Can you work these out from the model? Positions are in its coordinate system, mm. Face numbers are marked on the shaded views. A direction names the side the tool comes from. Round coordinates to 2 decimals unless told otherwise and drop trailing zeros. Order: outer loops, then holes, each group sorted by start corner. A loop starts at its lowest first (then second) coordinate and runs counter-clockwise, first axis right, second up. Notation, with made-up numbers: M 22,51 L 70,51 A25 ccw 70,84 Z; hole C -4,-35.75 d9. An arc over 180 degrees is marked long. One line per question, with ' | ' between items.
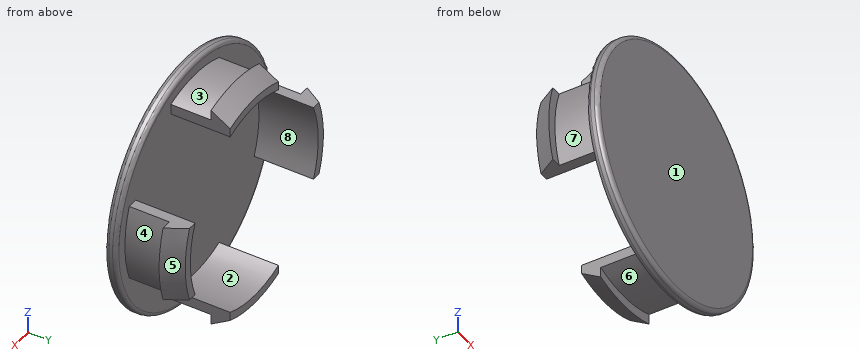
```python
from build123d import *

# Parameters (mm, degrees)
CUT_EXTRUDE_1_REACH = 51.545


with BuildPart() as part:
    # Эскиз1 → Повернуть1 (revolve)
    with BuildSketch(Plane.XY, mode=Mode.PRIVATE) as revolve_1_sk:
        with BuildLine():
            Line((0, 0), (-31.5, 0))
            ThreePointArc((-31.5, 0), (-32.207106781, 0.292893219), (-32.5, 1))
            Line((-32.5, 1), (-32.5, 2))
            ThreePointArc((-32.5, 2), (-32.207106781, 2.707106781), (-31.5, 3))
            Line((-31.5, 3), (-29, 3))
            Line((-29, 3), (-29, 13.5))
            Line((-29, 13.5), (-31.5, 13.5))
            Line((-31.5, 13.5), (-28.613248654, 18.5))
            Line((-28.613248654, 18.5), (-26.5, 18.5))
            Line((-26.5, 18.5), (-26.5, 3))
            Line((-26.5, 3), (0, 3))
            Line((0, 3), (0, 0))
        make_face()
    revolve(revolve_1_sk.sketch.rotate(Axis((0, 0, 0), (0, -1, 0)), 270), axis=Axis((0, 0, 0), (0, -1, 0)))

    # Вырез-Вытянуть1: up to this face of the body (flat: up to its plane)
    cut_extrude_1_end = Plane(part.part.faces().sort_by_distance((0, 3, -30.609045456))[0])
    # Эскиз2 → Вырез-Вытянуть1 (cut, up to the picked face)
    with BuildSketch(Plane(origin=(0, 18.5, 0), x_dir=(1, 0, 0), z_dir=(0, 1, 0)), mode=Mode.PRIVATE) as cut_extrude_1_sk1:
        with BuildLine():
            Line((-10, 26.8089164), (-10, 40.856644609))
            ThreePointArc((-10, 40.856644609), (-29.742775667, 29.742775667), (-40.856644609, 10))
            Line((-40.856644609, 10), (-26.8089164, 10))
            ThreePointArc((-26.8089164, 10), (-20.232622155, 20.232622155), (-10, 26.8089164))
        make_face()
    cut_extrude_1_tool1 = split(extrude(cut_extrude_1_sk1.sketch, amount=-CUT_EXTRUDE_1_REACH, mode=Mode.PRIVATE), bisect_by=cut_extrude_1_end, keep=Keep.BOTH, mode=Mode.PRIVATE)
    # Эскиз2 → Вырез-Вытянуть1 (cut, up to the picked face)
    with BuildSketch(Plane(origin=(0, 18.5, 0), x_dir=(1, 0, 0), z_dir=(0, 1, 0)), mode=Mode.PRIVATE) as cut_extrude_1_sk2:
        with BuildLine():
            ThreePointArc((26.8089164, 10), (20.232622155, 20.232622155), (10, 26.8089164))
            Line((10, 26.8089164), (10, 24.540782384))
            ThreePointArc((10, 24.540782384), (18.738329701, 18.738329701), (24.540782384, 10))
            Line((24.540782384, 10), (26.8089164, 10))
        make_face()
    cut_extrude_1_tool2 = split(extrude(cut_extrude_1_sk2.sketch, amount=-CUT_EXTRUDE_1_REACH, mode=Mode.PRIVATE), bisect_by=cut_extrude_1_end, keep=Keep.BOTH, mode=Mode.PRIVATE)
    # Эскиз2 → Вырез-Вытянуть1 (cut, up to the picked face)
    with BuildSketch(Plane(origin=(0, 18.5, 0), x_dir=(1, 0, 0), z_dir=(0, 1, 0)), mode=Mode.PRIVATE) as cut_extrude_1_sk3:
        with BuildLine():
            ThreePointArc((40.856644609, 10), (29.742775667, 29.742775667), (10, 40.856644609))
            Line((10, 40.856644609), (10, 26.8089164))
            ThreePointArc((10, 26.8089164), (20.232622155, 20.232622155), (26.8089164, 10))
            Line((26.8089164, 10), (40.856644609, 10))
        make_face()
    cut_extrude_1_tool3 = split(extrude(cut_extrude_1_sk3.sketch, amount=-CUT_EXTRUDE_1_REACH, mode=Mode.PRIVATE), bisect_by=cut_extrude_1_end, keep=Keep.BOTH, mode=Mode.PRIVATE)
    # Эскиз2 → Вырез-Вытянуть1 (cut, up to the picked face)
    with BuildSketch(Plane(origin=(0, 18.5, 0), x_dir=(1, 0, 0), z_dir=(0, 1, 0)), mode=Mode.PRIVATE) as cut_extrude_1_sk4:
        with BuildLine():
            ThreePointArc((10, -40.856644609), (29.742775667, -29.742775667), (40.856644609, -10))
            Line((40.856644609, -10), (26.8089164, -10))
            ThreePointArc((26.8089164, -10), (20.232622155, -20.232622155), (10, -26.8089164))
            Line((10, -26.8089164), (10, -40.856644609))
        make_face()
    cut_extrude_1_tool4 = split(extrude(cut_extrude_1_sk4.sketch, amount=-CUT_EXTRUDE_1_REACH, mode=Mode.PRIVATE), bisect_by=cut_extrude_1_end, keep=Keep.BOTH, mode=Mode.PRIVATE)
    # Эскиз2 → Вырез-Вытянуть1 (cut, up to the picked face)
    with BuildSketch(Plane(origin=(0, 18.5, 0), x_dir=(1, 0, 0), z_dir=(0, 1, 0)), mode=Mode.PRIVATE) as cut_extrude_1_sk5:
        with BuildLine():
            ThreePointArc((10, -26.8089164), (20.232622155, -20.232622155), (26.8089164, -10))
            Line((26.8089164, -10), (24.540782384, -10))
            ThreePointArc((24.540782384, -10), (18.738329701, -18.738329701), (10, -24.540782384))
            Line((10, -24.540782384), (10, -26.8089164))
        make_face()
    cut_extrude_1_tool5 = split(extrude(cut_extrude_1_sk5.sketch, amount=-CUT_EXTRUDE_1_REACH, mode=Mode.PRIVATE), bisect_by=cut_extrude_1_end, keep=Keep.BOTH, mode=Mode.PRIVATE)
    # Эскиз2 → Вырез-Вытянуть1 (cut, up to the picked face)
    with BuildSketch(Plane(origin=(0, 18.5, 0), x_dir=(1, 0, 0), z_dir=(0, 1, 0)), mode=Mode.PRIVATE) as cut_extrude_1_sk6:
        with BuildLine():
            Line((-26.8089164, -10), (-40.856644609, -10))
            ThreePointArc((-40.856644609, -10), (-29.742775667, -29.742775667), (-10, -40.856644609))
            Line((-10, -40.856644609), (-10, -26.8089164))
            ThreePointArc((-10, -26.8089164), (-20.232622155, -20.232622155), (-26.8089164, -10))
        make_face()
    cut_extrude_1_tool6 = split(extrude(cut_extrude_1_sk6.sketch, amount=-CUT_EXTRUDE_1_REACH, mode=Mode.PRIVATE), bisect_by=cut_extrude_1_end, keep=Keep.BOTH, mode=Mode.PRIVATE)
    # Эскиз2 → Вырез-Вытянуть1 (cut, up to the picked face)
    with BuildSketch(Plane(origin=(0, 18.5, 0), x_dir=(1, 0, 0), z_dir=(0, 1, 0)), mode=Mode.PRIVATE) as cut_extrude_1_sk7:
        with BuildLine():
            Line((-24.540782384, -10), (-26.8089164, -10))
            ThreePointArc((-26.8089164, -10), (-20.232622155, -20.232622155), (-10, -26.8089164))
            Line((-10, -26.8089164), (-10, -24.540782384))
            ThreePointArc((-10, -24.540782384), (-18.738329701, -18.738329701), (-24.540782384, -10))
        make_face()
    cut_extrude_1_tool7 = split(extrude(cut_extrude_1_sk7.sketch, amount=-CUT_EXTRUDE_1_REACH, mode=Mode.PRIVATE), bisect_by=cut_extrude_1_end, keep=Keep.BOTH, mode=Mode.PRIVATE)
    # Эскиз2 → Вырез-Вытянуть1 (cut, up to the picked face)
    with BuildSketch(Plane(origin=(0, 18.5, 0), x_dir=(1, 0, 0), z_dir=(0, 1, 0)), mode=Mode.PRIVATE) as cut_extrude_1_sk8:
        with BuildLine():
            Line((-10, 24.540782384), (-10, 26.8089164))
            ThreePointArc((-10, 26.8089164), (-20.232622155, 20.232622155), (-26.8089164, 10))
            Line((-26.8089164, 10), (-24.540782384, 10))
            ThreePointArc((-24.540782384, 10), (-18.738329701, 18.738329701), (-10, 24.540782384))
        make_face()
    cut_extrude_1_tool8 = split(extrude(cut_extrude_1_sk8.sketch, amount=-CUT_EXTRUDE_1_REACH, mode=Mode.PRIVATE), bisect_by=cut_extrude_1_end, keep=Keep.BOTH, mode=Mode.PRIVATE)
    add(cut_extrude_1_tool1.solids().sort_by(Axis((-24.400112, 18.5, -24.400112), (0, -1, 0)))[0], mode=Mode.SUBTRACT)
    add(cut_extrude_1_tool2.solids().sort_by(Axis((18.950359, 18.5, -18.950359), (0, -1, 0)))[0], mode=Mode.SUBTRACT)
    add(cut_extrude_1_tool3.solids().sort_by(Axis((24.400112, 18.5, -24.400112), (0, -1, 0)))[0], mode=Mode.SUBTRACT)
    add(cut_extrude_1_tool4.solids().sort_by(Axis((24.400112, 18.5, 24.400112), (0, -1, 0)))[0], mode=Mode.SUBTRACT)
    add(cut_extrude_1_tool5.solids().sort_by(Axis((18.950359, 18.5, 18.950359), (0, -1, 0)))[0], mode=Mode.SUBTRACT)
    add(cut_extrude_1_tool6.solids().sort_by(Axis((-24.400112, 18.5, 24.400112), (0, -1, 0)))[0], mode=Mode.SUBTRACT)
    add(cut_extrude_1_tool7.solids().sort_by(Axis((-18.950359, 18.5, 18.950359), (0, -1, 0)))[0], mode=Mode.SUBTRACT)
    add(cut_extrude_1_tool8.solids().sort_by(Axis((-18.950359, 18.5, -18.950359), (0, -1, 0)))[0], mode=Mode.SUBTRACT)


solid = part.part
```
(1) On a 3-axis mill with a long thin cutter (end or side, diameter ignored), from which of +Z, -Z, +X, -X, +Y, -Y can I reach the whole of each face in a straight line? I mean the marked faces 4, 5, 6, 7 and 8. Say none if no direction works.
Final values:
face 4: +X | face 5: +X, +Y | face 6: -Z | face 7: -X | face 8: +Y
(2) If we section it at C-C on x = 0: Please give me the cut outline in (y, z).
Final values:
outline: M 0,-31.5 A1 ccw 1,-32.5 L 2,-32.5 A1 ccw 3,-31.5 L 3,-29 L 13.5,-29 L 13.5,-31.5 L 18.5,-28.61 L 18.5,-26.5 L 3,-26.5 L 3,26.5 L 18.5,26.5 L 18.5,28.61 L 13.5,31.5 L 13.5,29 L 3,29 L 3,31.5 A1 ccw 2,32.5 L 1,32.5 A1 ccw 0,31.5 Z
(3) Please list where these lines run through material, in increasing order: probe 1 along Y at (x, z) = (-28, -14); probe 2 along Z at (x, y) = (8, 9); probe 3 along Z at (x, y) = (5, 15). Write a range as [from, to].
Final values:
probe 1: [0, 3] | probe 2: [-27.87, -25.26], [25.26, 27.87] | probe 3: [-30.22, -26.02], [26.02, 30.22]
(4) Will these pins go through, and if not, where does the flat tip stop? pin 1 Ø5 at (y, z) = (4.5, 0) entering from -X; pin 2 Ø3 at (x, z) = (9, 13) entering from +Y; pin 3 Ø1.6 at (x, y) = (28.5, 14) entering from +Z.
Final values:
pin 1: x = -32.5 | pin 2: y = 3 | pin 3: z = 10
(5) Thinking about a two-plate mould opening in X: for the marked faces 1, 2 and 3, which applies, released by +X, released by -X, zero draft, split by the parting line, or undercut?
Final values:
face 1: zero draft | face 2: undercut | face 3: split by the parting line
(6) If we section it at B-B on z = 0: Please give me the cut outline in (x, y).
Final values:
outline: M -32.5,1 A1 ccw -31.5,0 L 31.5,0 A1 ccw 32.5,1 L 32.5,2 A1 ccw 31.5,3 L 29,3 L 29,13.5 L 31.5,13.5 L 28.61,18.5 L 26.5,18.5 L 26.5,3 L -26.5,3 L -26.5,18.5 L -28.61,18.5 L -31.5,13.5 L -29,13.5 L -29,3 L -31.5,3 A1 ccw -32.5,2 Z
(7) If we section it at A-A on y = 5.5: Please give me the cut outline in (x, z).
Final values:
outline: M -27.22,-10 L -24.54,-10 A26.5 cw -24.54,10 L -27.22,10 A29 ccw Z; M -10,-27.22 A29 ccw 10,-27.22 L 10,-24.54 A26.5 cw -10,-24.54 Z; M -10,24.54 A26.5 cw 10,24.54 L 10,27.22 A29 ccw -10,27.22 Z; M 24.54,-10 L 27.22,-10 A29 ccw 27.22,10 L 24.54,10 A26.5 cw Z
